```python
from build123d import *

# Parameters (mm, degrees)
SKETCH_1_W      = 600
SKETCH_1_H      = 600
EXTRUDE_1_DEPTH = 1700
SKETCH_2_W      = 650
SKETCH_2_H      = 50
EXTRUDE_2_DEPTH = 1700
SKETCH_3_W      = 50
SKETCH_3_H      = 100
EXTRUDE_3_DEPTH = 800
SKETCH_4_W      = 700
SKETCH_4_H      = 700
EXTRUDE_4_DEPTH = 50


with BuildPart() as part:
    # 草图1 → 凸台-拉伸1 (new body)
    with BuildSketch(Plane.XY):
        Rectangle(SKETCH_1_W, SKETCH_1_H)
    extrude(amount=EXTRUDE_1_DEPTH)

    # 草图2 → 凸台-拉伸2 (add)
    with BuildSketch(Plane.XY):
        with Locations((0, 325)):
            Rectangle(SKETCH_2_W, SKETCH_2_H)
    extrude(amount=EXTRUDE_2_DEPTH)

    # 草图3 → 凸台-拉伸3 (add)
    with BuildSketch(Plane.XY):
        with Locations((325, 0)):
            Rectangle(SKETCH_3_W, SKETCH_3_H)
    extrude(amount=EXTRUDE_3_DEPTH)

    # 草图4 → 凸台-拉伸4 (add)
    with BuildSketch(Plane.XY):
        Rectangle(SKETCH_4_W, SKETCH_4_H)
    extrude(amount=EXTRUDE_4_DEPTH)


solid = part.part
```
Input: part model. Units: mm. Frame: model coordinates. A direction names the side the tool comes from. Give positions to 0.01 mm unless a question says otherwise; leave off trailing zeros. Loops run counter-clockwise (first coordinate to the right, second up) from the corner with the lowest first, then second, coordinate; pieces in that order, holes last. Notation, with made-up numbers: (59.5, 80.25) -> (71.5, 80.25) arc R33 cw to (71.5, 118.25) -> close; hole circle Ø3 at (-6, 22). An arc over 180 degrees is marked (long way). Use a Markdown table: item, result.
Q1. Ray query, probe 1 along X at (y, z) = (318.5, 659); probe 2 along Y at (x, z) = (-260, 483.5); probe 3 along Y at (x, z) = (-305, 411). Return the intervals inside material, ascending. Write a range as from..to.
Entries:
| item | result |
|---|---|
| probe 1 | x = -325..325 |
| probe 2 | y = -300..350 |
| probe 3 | y = 300..350 |
Q2. Section query C-C, the plane x = -184. Return the cut outline in (y, z).
Entries:
| item | result |
|---|---|
| outline | (-350, 0) -> (350, 0) -> (350, 1700) -> (-300, 1700) -> (-300, 50) -> (-350, 50) -> close |
Q3. Pull-direction query (Y, two-part tool) for faces 6 (the flat face through (-79, -309, 50)), 7 (the flat face through (300, -4, 863)), 8 (the flat face through (-4, -300, 863)); classes: pulls with the +Y half, pulls with the -Y half, needs draft (parallel to the pull), parting line crosses it, or undercut.
Entries:
| item | result |
|---|---|
| face 6 | needs draft |
| face 7 | undercut |
| face 8 | pulls with the -Y half |
Q4. Access query for faces 1 (the flat face through (325, 1, 800)), 2 (the flat face through (-300, -4, 863)), 3 (the flat face through (-325, 325, 863)), 4 (the flat face through (325, 325, 863)), 5 (the flat face through (325, 50, 420)). Directions: +Z, -Z, +X, -X, +Y, -Y. A direction counts if a zero-diameter tool reaches every point of the face in a straight line with its end or side. Return the directions, or none.
Entries:
| item | result |
|---|---|
| face 1 | +Z, +X, -Y |
| face 2 | +Z, -X, -Y |
| face 3 | +Z, -X, +Y, -Y |
| face 4 | +Z, +X, +Y |
| face 5 | +Z, +X |
Q5. Section query D-D, the plane z = 199. Return the cut outline in (x, y), plus the area to 4 significant figures.
Entries:
| item | result |
|---|---|
| outline | (-325, 300) -> (-300, 300) -> (-300, -300) -> (300, -300) -> (300, -50) -> (350, -50) -> (350, 50) -> (300, 50) -> (300, 300) -> (325, 300) -> (325, 350) -> (-325, 350) -> close |
| area | 397,500 mm² |
Q6. Section query B-B, the plane z = 963.5. Return the cut outline in (x, y), plus the area to 4 significant figures.
Entries:
| item | result |
|---|---|
| outline | (-325, 300) -> (-300, 300) -> (-300, -300) -> (300, -300) -> (300, 300) -> (325, 300) -> (325, 350) -> (-325, 350) -> close |
| area | 392,500 mm² |
Q7. Section query A-A, the plane y = -167. Return the cut outline in (x, z), plus the area to 4 significant figures.
Entries:
| item | result |
|---|---|
| outline | (-350, 0) -> (350, 0) -> (350, 50) -> (300, 50) -> (300, 1700) -> (-300, 1700) -> (-300, 50) -> (-350, 50) -> close |
| area | 1,025,000 mm² |
Q8. First-contact query: P1, Ø2, axis at y = 38.5, z = 857, coming from the -X side; P2, Ø6, axis at y = 162.5, z = 1142.5, coming from the +X side; P3, Ø25, axis at x = 320, z = 291, coming from the -Y side. Flat tips, straight axial feed; report the tip coordinate or a pass-through.
Entries:
| item | result |
|---|---|
| P1 | stops at x = -300 |
| P2 | stops at x = 300 |
| P3 | stops at y = -50 |
